For this review, take the finished solid that the model builds, in its own axes (mm). Face numbers are marked on the shaded views. A direction names the side the tool comes from. Round coordinates to 2 decimals unless told otherwise and drop trailing zeros. Write each loop counter-clockwise with the first axis right and the second up, starting at its lowest first coordinate (ties: lowest second). Pieces come first, ordered by that corner, then holes.
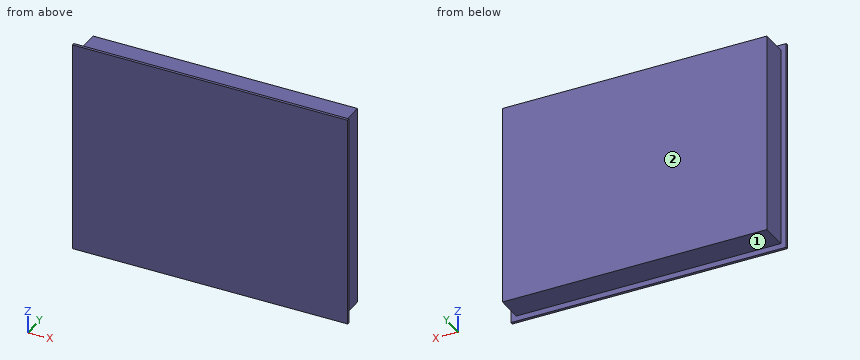
from build123d import *

# Parameters (mm, degrees)
F1_W     = 298
F1_H     = 228
F2_DEPTH = 30
F0_W     = 310
F0_H     = 240
F3_DEPTH = 3


with BuildPart() as f2:
    # F1 (on face) → F2 (new body)
    with BuildSketch(Plane.XZ):
        Rectangle(F1_W, F1_H)
    extrude(amount=-F2_DEPTH)

    # F0 (on Front) → F3 (join)
    with BuildSketch(Plane.XZ):
        Rectangle(F0_W, F0_H)
    extrude(amount=F3_DEPTH)


solid = f2.part
(1) We need section B-B, the plane z = 77.5. Give the boundary of the cut face in (x, y).
Geometry check:
outline: (-155, -3) - (155, -3) - (155, 0) - (149, 0) - (149, 30) - (-149, 30) - (-149, 0) - (-155, 0) - close
(2) For line 1 along Z through (x, y) = (26, 5); line 2 along X through (y, z) = (10, -3.5), list the stretches that pass through material, from the lowest coordinate up.
Geometry check:
line 1: z = -114 to 114
line 2: x = -149 to 149
(3) For the marked faces 1 and 2, list the 3-axis set-ups (+Z, -Z, +X, -X, +Y, -Y) from which the entire face can be reached by the end or side of a thin tool; tool diameter is ignored.
Geometry check:
face 1: -Z, +X, -X, +Y
face 2: +Z, -Z, +X, -X, +Y
(4) We need section A-A, the plane x = 35. Give the boundary of the cut face in (y, z).
Geometry check:
outline: (-3, -120) - (0, -120) - (0, -114) - (30, -114) - (30, 114) - (0, 114) - (0, 120) - (-3, 120) - close
(5) We need section C-C, the plane y = 7. Give the boundary of the cut face in (x, z), and give its area (3 significant figures).
Geometry check:
outline: (-149, -114) - (149, -114) - (149, 114) - (-149, 114) - close
area: 67,900 mm2
(6) For pin 1 Ø10 at (x, y) = (48.5, 8.5) entering from +Z; pin 2 Ø3 at (x, y) = (67, 15) entering from -Z; pin 3 Ø6 at (y, z) = (6, 81.5) entering from +X, all flat-tipped, find the tip position at first contact; note any pin that passes through.
Geometry check:
pin 1: stops at z = 114
pin 2: stops at z = -114
pin 3: stops at x = 149
